```python
from build123d import *

# Parameters (mm, degrees)
SKETCH1_R           = 10.25
SKETCH1_R_2         = 4.14
BOSS_EXTRUDE1_DEPTH = 10
CHAMFER1_SIZE       = 0.5
CUT_EXTRUDE1_DEPTH  = 15.5


with BuildPart() as part:
    # Sketch1 → Boss-Extrude1 (new, symmetric)
    with BuildSketch(Plane.XY):
        with BuildLine():
            Line((-7.444896481, 30.480652594), (-29.444896481, 30.480652594))
            ThreePointArc((-29.444896481, 30.480652594), (-36.515964293, 27.551720406), (-39.444896481, 20.480652594))
            Line((-39.444896481, 20.480652594), (-39.444896481, -31.519347406))
            Line((-39.444896481, -31.519347406), (2.555103519, -31.519347406))
            Line((2.555103519, -31.519347406), (2.555103519, 20.480652594))
            ThreePointArc((2.555103519, 20.480652594), (-0.373828669, 27.551720406), (-7.444896481, 30.480652594))
        make_face()
        with Locations((-18.444896481, 9.480652594)):
            Circle(SKETCH1_R, mode=Mode.SUBTRACT)
        with Locations((-18.444896481, -11.019347406)):
            Circle(SKETCH1_R_2, mode=Mode.SUBTRACT)
    extrude(amount=BOSS_EXTRUDE1_DEPTH, both=True)

    # Chamfer1
    chamfer1_edges = [part.edges().sort_by_distance(p)[0] for p in [
        (-22.584896481, -11.019347406, -10),
        (-22.584896481, -11.019347406, 10),
        (-28.694896481, 9.480652594, -10),
        (-28.694896481, 9.480652594, 10),
    ]]
    chamfer(chamfer1_edges, length=CHAMFER1_SIZE)

    # Sketch3 → Cut-Extrude1 (cut)
    with BuildSketch(Plane(origin=(0, -31.519347406, 0), x_dir=(-1, 0, 0), z_dir=(0, -1, 0))):
        Polygon((33.444896481, -3.25), (36.259479043, -1.625), (36.259479043, 1.625), (33.444896481, 3.25), (30.630313919, 1.625), (30.630313919, -1.625), align=None)
    cut_extrude1 = extrude(amount=-CUT_EXTRUDE1_DEPTH, mode=Mode.SUBTRACT)

    # Mirror1: Cut-Extrude1 across plane
    add(cut_extrude1.mirror(Plane(origin=(-18.444896481, 0, 0), x_dir=(0, 0, 1), z_dir=(1, 0, 0))), mode=Mode.SUBTRACT)


solid = part.part
```
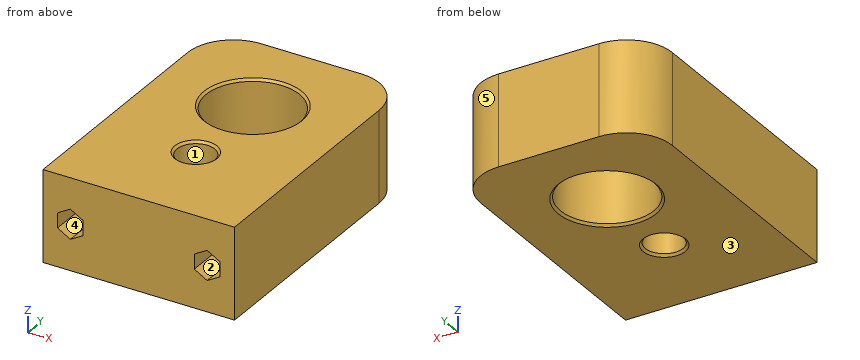
Check sheet for the modelled part. Datum: model origin and axes. Units: mm. Face numbers are marked on the shaded views. A direction names the side the tool comes from. Give positions to 0.01 mm unless a question says otherwise; leave off trailing zeros. Write each loop counter-clockwise with the first axis right and the second up, starting at its lowest first coordinate (ties: lowest second). Pieces come first, ordered by that corner, then holes. Notation, with made-up numbers: (85, 64) - (120, 64) arc R23 ccw to (120, 97) - close; hole circle Ø2 at (84.25, 40.25). An arc over 180 degrees is marked (long way). Answer as a JSON object with one key per item and string values. Group by question number.
1) Sectioned sample at B-B (z = -6.5). Record the cut outline in (x, y), then the cut area to 3 significant figures.
2) Sectioned sample at C-C (x = -35). Record the cut outline in (y, z).
3) Thickness scan on probe 1 along X at (y, z) = (10, 3); probe 2 along Y at (x, z) = (-17, -4.25); probe 3 along Y at (x, z) = (-22, 8.25). Record the ranges inside material, lowest first. Write a range as from..to.
4) Access from +Z, -Z, +X, -X, +Y, -Y to the whole of each face (thin tool, end or side, straight path). Record for the marked faces 4 and 5.
5) Sectioned sample at A-A (y = -20.5). Record the cut outline in (x, z) (3 decimals), then the cut area to 3 significant figures.
6) Depth check by flat-ended pin: P1, Ø18.5, axis at x = -18.44, y = 9.48, coming from the +Z side; P2, Ø6, axis at x = -32.5, z = 0.5, coming from the -Y side; P3, Ø1.7, axis at x = -3, z = 0.5, coming from the -Y side. Enter the tip coordinate at first touch or a pass-through.
7) Release check for a two-part mould opening along Z. For the marked faces 1, 2 and 3 record: pulls with the +Z half, pulls with the -Z half, needs draft (parallel to the pull), parting line crosses it, or undercut.
8) Sectioned sample at D-D (x = -15.5). Give the number of separate pieces and of enclosed holes in the cut face, then the cut area to 3 significant figures.
Geometry results:
{
 "1": {"outline": "(-39.44, -31.52) - (2.56, -31.52) - (2.56, 20.48) arc R10 ccw to (-7.44, 30.48) - (-29.44, 30.48) arc R10 ccw to (-39.44, 20.48) - close; hole circle Ø20.5 at (-18.44, 9.48); hole circle Ø8.28 at (-18.44, -11.02)", "area": "2,180 mm^2"},
 "2": {"outline": "(-31.52, -10) - (28.8, -10) - (28.8, 10) - (-31.52, 10) - (-31.52, 2.35) - (-16.02, 2.35) - (-16.02, -2.35) - (-31.52, -2.35) - close"},
 "3": {"probe 1": "x = -39.44..-28.68, -8.21..2.56", "probe 2": "y = -31.52..-14.9, -7.14..-0.67, 19.63..30.48", "probe 3": "y = -31.52..-13.14, -8.9..-0.13, 19.09..30.48"},
 "4": {"face 4": "-Y", "face 5": "+Z, -Z, +X, +Y"},
 "5": {"outline": "(-39.445, -10) - (2.555, -10) - (2.555, 10) - (-39.445, 10) - close; hole (-36.259, -1.625) - (-33.445, -3.25) - (-30.63, -1.625) - (-30.63, 1.625) - (-33.445, 3.25) - (-36.259, 1.625) - close; hole (-6.259, -1.625) - (-3.445, -3.25) - (-0.63, -1.625) - (-0.63, 1.625) - (-3.445, 3.25) - (-6.259, 1.625) - close", "area": "785 mm^2"},
 "6": {"P1": "passes through", "P2": "stops at y = -31.52", "P3": "stops at y = -16.02"},
 "7": {"face 1": "needs draft", "face 2": "undercut", "face 3": "pulls with the -Z half"},
 "8": {"separate pieces": "3", "enclosed holes": "0", "area": "730 mm^2"}
}
